Design review of the part built by this model. Coordinates are the model's own, in mm. Face numbers are marked on the shaded views. A direction names the side the tool comes from. Give positions to 0.01 mm unless a question says otherwise; leave off trailing zeros. Write each loop counter-clockwise with the first axis right and the second up, starting at its lowest first coordinate (ties: lowest second). Pieces come first, ordered by that corner, then holes.
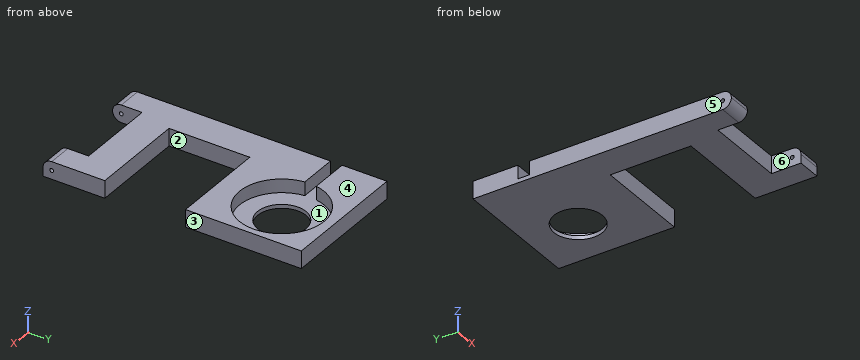
```python
from build123d import *

# Parameters (mm, degrees)
F0_W      = 50.8
F0_H      = 101.6
F1_DEPTH  = 6.858
F2_R      = 16.637
F3_DEPTH  = 5.334
F4_R      = 9.525
F5_DEPTH  = 25.4
F6_W      = 31.75
F6_H      = 11.6078
F7_DEPTH  = 25.4
F8_W      = 38.1
F8_H      = 31.75
F9_DEPTH  = 25.4
F10_R     = 3.42899
F12_DEPTH = 5.334
F13_R     = 0.762
F14_DEPTH = 50.8


# Not quite as in the source:
# - a fillet or chamfer is up to 0.001 mm smaller than in the source, because OpenCascade refuses the exact size


with BuildPart() as f1:
    # F0 (on Top) → F1 (new body)
    with BuildSketch(Plane.XY):
        with Locations((6.0819597751, 21.255746996)):
            Rectangle(F0_W, F0_H)
    extrude(amount=F1_DEPTH)

    # F2 (on face) → F3 (cut)
    with BuildSketch(Plane.XY.offset(6.858)):
        with Locations((12.4319597751, 51.735746996)):
            Circle(F2_R)
    extrude(amount=-F3_DEPTH, mode=Mode.SUBTRACT)

    # F4 (on face) → F5 (cut)
    with BuildSketch(Plane.XY.offset(1.524)):
        with Locations((12.4319597751, 51.735746996)):
            Circle(F4_R)
    extrude(amount=-F5_DEPTH, mode=Mode.SUBTRACT)

    # F6 (on face) → F7 (cut)
    with BuildSketch(Plane.XY.offset(6.858)):
        with Locations((6.0819597751, -23.740353004)):
            Rectangle(F6_W, F6_H)
    extrude(amount=-F7_DEPTH, mode=Mode.SUBTRACT)

    # F8 (on face) → F9 (cut)
    with BuildSketch(Plane.XY.offset(6.858)):
        with Locations((12.4319597751, 10.638546996)):
            Rectangle(F8_W, F8_H)
    extrude(amount=-F9_DEPTH, mode=Mode.SUBTRACT)

    # F10 (radius 3.429 in the source; OpenCascade refuses exactly that, so slightly less here)
    f10_edges = [f1.edges().sort_by_distance(p)[0] for p in [
        (-14.55554, -29.544253, 6.858),
        (26.71946, -29.544253, 6.858),
        (-14.55554, -29.544253, 0),
    ]]
    fillet(f10_edges, radius=F10_R)

    # F11 (on face) → F12 (cut)
    with BuildSketch(Plane.XY.offset(6.858)):
        with BuildLine():
            Line((-3.9898817782, 54.402746996), (-19.3180402249, 54.402746996))
            Line((-19.3180402249, 54.402746996), (-19.3180402249, 49.830746996))
            Line((-19.3180402249, 49.830746996), (-4.0956154857, 49.830746996))
            ThreePointArc((-4.0956154857, 49.830746996), (-4.2005930385, 52.1203973622), (-3.9898817782, 54.402746996))
        make_face()
    extrude(amount=-F12_DEPTH, mode=Mode.SUBTRACT)

    # F13 (on face) → F14 (cut)
    with BuildSketch(Plane(origin=(-19.3180402249, 0, 0), x_dir=(0, -1, 0), z_dir=(-1, 0, 0))):
        with Locations((26.115253004, 3.429)):
            Circle(F13_R)
    extrude(amount=-F14_DEPTH, mode=Mode.SUBTRACT)


solid = f1.part
```
(1) Mouldability with a two-part tool opening along X and no side actions: class the marked faces 4, 5 and 6 as pulls with the +X half, pulls with the -X half, needs draft (parallel to the pull), parting line crosses it, or undercut.
Resolved:
face 4: needs draft
face 5: pulls with the -X half
face 6: undercut
(2) Consider section C-C, the plane x = 26.5. Give the boundary of the cut face in (y, z), then the cut area to 3 significant figures.
Resolved:
outline: (-29.54, 0) - (-5.24, 0) - (-5.24, 6.86) - (-26.12, 6.86) arc R3.43 ccw to (-29.54, 3.43) - close; (26.51, 0) - (72.06, 0) - (72.06, 6.86) - (60.62, 6.86) - (60.62, 1.52) - (42.85, 1.52) - (42.85, 6.86) - (26.51, 6.86) - close; hole circle Ø1.52 at (-26.12, 3.43)
area: 380 mm2
(3) Consider section A-A, the plane x = 14.5. Give the boundary of the cut face in (y, z), then the cut area to 3 significant figures.
Resolved:
outline: (-17.94, 0) - (-5.24, 0) - (-5.24, 6.86) - (-17.94, 6.86) - close; (26.51, 0) - (42.44, 0) - (42.44, 1.52) - (35.23, 1.52) - (35.23, 6.86) - (26.51, 6.86) - close; (61.03, 0) - (72.06, 0) - (72.06, 6.86) - (68.24, 6.86) - (68.24, 1.52) - (61.03, 1.52) - close
area: 195 mm2
(4) Clearance check with a flat-ended pin moving along its axis: P1, Ø3.5, axis at x = 14, z = 5, coming from the -Y side. State where the tip first meets the part, or that it passes through.
Resolved:
P1: stops at y = -17.94
(5) Consider section B-B, the plane y = 60. Give the boundary of the cut face in (x, z).
Resolved:
outline: (-19.32, 0) - (7.7, 0) - (7.7, 1.52) - (-2.01, 1.52) - (-2.01, 6.86) - (-19.32, 6.86) - close; (17.17, 0) - (31.48, 0) - (31.48, 6.86) - (26.87, 6.86) - (26.87, 1.52) - (17.17, 1.52) - close
(6) To check wall thickness, follow L1, parallel to Y at x = 7.5, z = 1.25; L2, parallel to Y at x = 23, z = 2.5; L3, parallel to Y at x = 23, z = 3.5. State the ranges of each line that lie inside material, in increasing order.
Resolved:
L1: y = -17.94 to -5.24, 26.51 to 43.59, 59.88 to 72.06
L2: y = -29.54 to -5.24, 26.51 to 38.89, 64.59 to 72.06
L3: y = -29.54 to -26.87, -25.36 to -5.24, 26.51 to 38.89, 64.59 to 72.06
(7) Tool access review of the marked faces 1, 2 and 3: name each direction out of +Z, -Z, +X, -X, +Y, -Y from which nothing blocks a thin tool from reaching the whole face with its end or side.
Resolved:
face 1: +Z
face 2: +Z, -Z, +X
face 3: +Z, -Z, +X, +Y, -Y
